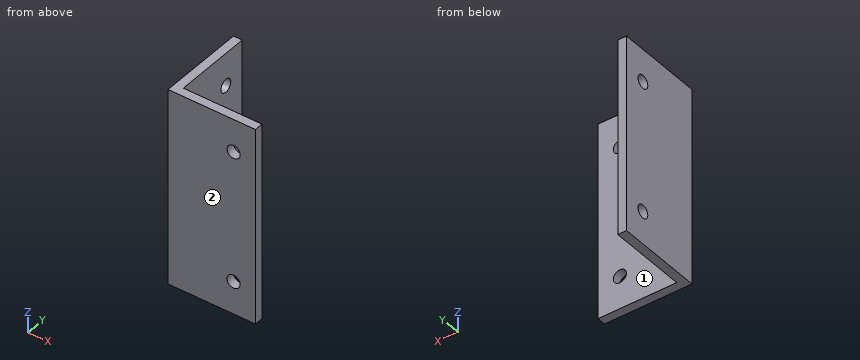
```python
from build123d import *

# Parameters (mm, degrees)
EXTRUDE_1_DEPTH     = 45
SKETCH_2_R          = 1.5
CUT_EXTRUDE_1_DEPTH = 52.701063819
SKETCH_3_R          = 1.5
CUT_EXTRUDE_2_DEPTH = 52.701063819


with BuildPart() as part:
    # 草图1 → 凸台-拉伸1 (new body)
    with BuildSketch(Plane.XY):
        Polygon((0, 0), (0, 18), (-2, 18), (-2, -2), (18, -2), (18, 0), align=None)
    extrude(amount=EXTRUDE_1_DEPTH)

    # 草图2 → 切除-拉伸1 (cut, through all)
    with BuildSketch(Plane(origin=(0, 0, 0), x_dir=(0, 0, -1), z_dir=(1, 0, 0))):
        with Locations((-37.5, 13)):
            Circle(SKETCH_2_R)
        with Locations(Location((-7.5, 13, 0), (0, 0, 180))):
            Circle(SKETCH_2_R)
    extrude(amount=-CUT_EXTRUDE_1_DEPTH, mode=Mode.SUBTRACT)

    # 草图3 → 切除-拉伸2 (cut, through all)
    with BuildSketch(Plane(origin=(0, 0, 0), x_dir=(1, 0, 0), z_dir=(0, 1, 0))):
        with Locations(Location((13, -37.5, 0), (0, 0, 180))):
            Circle(SKETCH_3_R)
        with Locations((13, -7.5)):
            Circle(SKETCH_3_R)
    extrude(amount=-CUT_EXTRUDE_2_DEPTH, mode=Mode.SUBTRACT)


solid = part.part
```
Geometry: final body of the model. Coordinates: model frame, mm. Face numbers are marked on the shaded views. A direction names the side the tool comes from. Round coordinates to 2 decimals unless told otherwise and drop trailing zeros. Order: outer loops, then holes, each group sorted by start corner. A loop starts at its lowest first (then second) coordinate and runs counter-clockwise, first axis right, second up. Notation, with made-up numbers: (84.25, 60.25) -> (96.25, 60.25) arc R20 cw to (96.25, 95.25) -> close; hole circle Ø9 at (-23, 54.5). An arc over 180 degrees is marked (long way). Use CSV: the item, a comma, the result in double quotes. Start each with the question number.
1) Section A-A (z = 37.5). Return the cut outline in (x, y), and give its area (3 significant figures).
2) First-contact query: pin 1 Ø4 at (x, z) = (4.5, 5.5) entering from +Y; pin 2 Ø5 at (y, z) = (14.5, 19) entering from +X; pin 3 Ø2.5 at (x, z) = (13, 7.5) entering from +Y; pin 4 Ø4 at (x, y) = (1, 14.5) entering from +Z. Flat tips, straight axial feed; report the tip coordinate or a pass-through.
3) Set-up query: the marked faces 1 and 2. Return all of +Z, -Z, +X, -X, +Y, -Y with unobstructed straight access to the full face (end or side cutting, diameter ignored); none if empty.
4) Section B-B (x = 13). Return the cut outline in (y, z), and give its area (3 significant figures).
5) Material intervals for line 1 along Z through (x, y) = (13, -0.85); line 2 along Y through (x, z) = (-0.8, 7.5), sorted ascending. Write a range as from..to.
6) Section D-D (x = 9.75). Return the cut outline in (y, z), and give its area (3 significant figures).
Returned:
1,outline,"(-2, -2) -> (11.5, -2) -> (11.5, 0) -> (0, 0) -> (0, 11.5) -> (-2, 11.5) -> close; (-2, 14.5) -> (0, 14.5) -> (0, 18) -> (-2, 18) -> close; (14.5, -2) -> (18, -2) -> (18, 0) -> (14.5, 0) -> close"
1,area,"64.0 mm²"
2,pin 1,"stops at y = 0"
2,pin 2,"stops at x = 0"
2,pin 3,"passes through"
2,pin 4,"stops at z = 45"
3,face 1,"+Z, -Z, +X, +Y"
3,face 2,"+Z, -Z, +X, -X, -Y"
4,outline,"(-2, 0) -> (0, 0) -> (0, 6) -> (-2, 6) -> close; (-2, 9) -> (0, 9) -> (0, 36) -> (-2, 36) -> close; (-2, 39) -> (0, 39) -> (0, 45) -> (-2, 45) -> close"
4,area,"78.0 mm²"
5,line 1,"z = 0..6, 9..36, 39..45"
5,line 2,"y = -2..11.5, 14.5..18"
6,outline,"(-2, 0) -> (0, 0) -> (0, 45) -> (-2, 45) -> close"
6,area,"90.0 mm²"
